Drawing for the job (mm, zero at the part's lowest x, y, z). Give positions to 0.01 mm unless a question says otherwise; leave off trailing zeros. Order: outer loops, then holes, each group sorted by start corner. A loop starts at its lowest first (then second) coordinate and runs counter-clockwise, first axis right, second up. Notation, with made-up numbers: (0.25, 46) - (35.25, 46) arc R20 ccw to (35.25, 57) - close; hole circle Ø6 at (-35.5, 70). An arc over 180 degrees is marked (long way). Use a Markdown table: item, result.
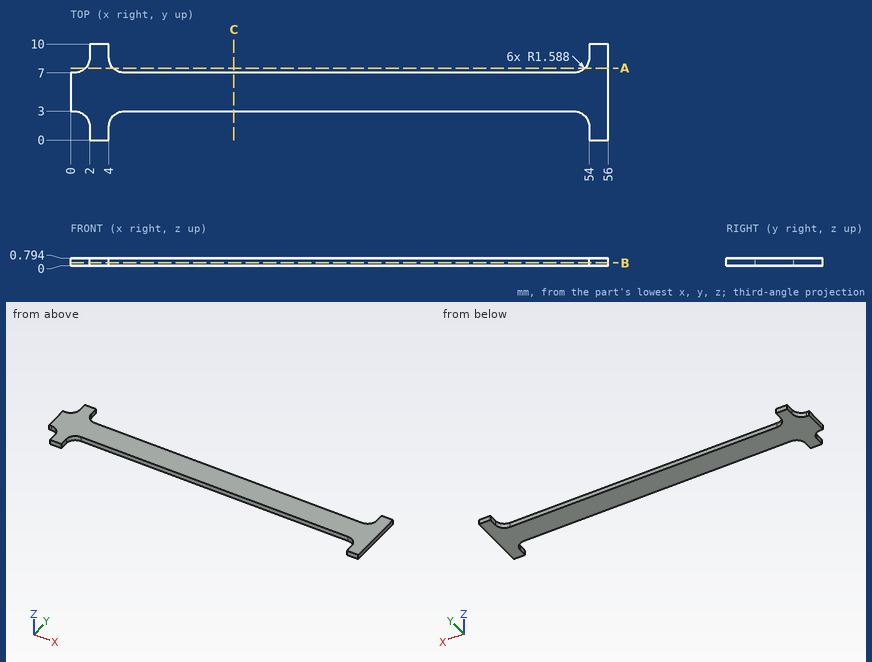
1) Wall check: line 1 (X direction, y = 9, z = 0.35); line 2 (Y direction, x = 18, z = 0.2); line 3 (X direction, y = 7.25, z = 0.35) (1 decimal). Give the ranges that are in metal, low to high. Write a range as from..to.
Computed:
| item | result |
|---|---|
| line 1 | x = 2..4, 54..56 |
| line 2 | y = 3..7 |
| line 3 | x = 1.3..4.7, 53.3..56 |
2) Slice it at C-C (x = 17). Write the cut outline in (y, z).
Computed:
| item | result |
|---|---|
| outline | (3, 0) - (7, 0) - (7, 0.79) - (3, 0.79) - close |
3) Slice it at B-B (z = 0.3). Write the cut outline in (x, y) (1 decimal), and give its area (3 significant figures).
Computed:
| item | result |
|---|---|
| outline | (0, 3) - (0.4, 3) arc R1.6 cw to (2, 1.4) - (2, 0) - (4, 0) - (4, 1.4) arc R1.6 cw to (5.6, 3) - (52.4, 3) arc R1.6 cw to (54, 1.4) - (54, 0) - (56, 0) - (56, 10) - (54, 10) - (54, 8.6) arc R1.6 cw to (52.4, 7) - (5.6, 7) arc R1.6 cw to (4, 8.6) - (4, 10) - (2, 10) - (2, 8.6) arc R1.6 cw to (0.4, 7) - (0, 7) - close |
| area | 251 mm² |
4) Slice it at A-A (y = 7.5). Write the cut outline in (x, z).
Computed:
| item | result |
|---|---|
| outline | (1.57, 0) - (4.43, 0) - (4.43, 0.79) - (1.57, 0.79) - close; (53.57, 0) - (56, 0) - (56, 0.79) - (53.57, 0.79) - close |
